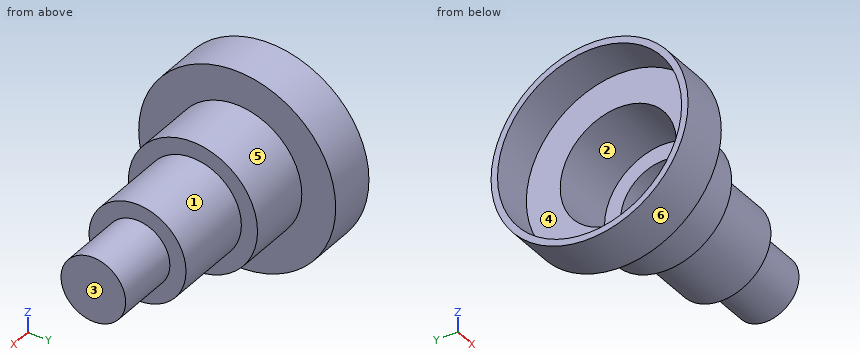
```python
from build123d import *

# Parameters (mm, degrees)
SVUOTA1_T = -2


with BuildPart() as part:
    # Schizzo1 → Rivoluzione1 (revolve)
    with BuildSketch(Plane.XY):
        Polygon((0, 0), (0, 30.5), (15, 30.5), (15, 20), (35, 20), (35, 15), (60, 15), (60, 10), (80, 10), (80, 0), align=None)
    revolve(axis=Axis((80, 0, 0), (-1, 0, 0)))

    # Svuota1
    svuota1_openings = [part.faces().sort_by_distance(p)[0] for p in [
        (0, 0, 0),
    ]]
    offset(amount=SVUOTA1_T, openings=svuota1_openings, kind=Kind.INTERSECTION)


solid = part.part
```
For this review, take the finished solid that the model builds, in its own axes (mm). Face numbers are marked on the shaded views. A direction names the side the tool comes from. Coordinates: 2 decimals unless noted, no trailing zeros. Order: outer loops, then holes, each group sorted by start corner. A loop starts at its lowest first (then second) coordinate and runs counter-clockwise, first axis right, second up. Notation, with made-up numbers: (-35, 27.25) - (13, 27.25) arc R21 cw to (13, 51.25) - close; hole circle Ø9 at (8, 29). An arc over 180 degrees is marked (long way). Answer as a JSON object with one key per item and string values. Group by question number.
1. We need section D-D on z = 11.5. State the section outline as (x, y) points, then the cut area to 3 significant figures.
2. For the marked faces 4, 5 and 6, list the 3-axis set-ups (+Z, -Z, +X, -X, +Y, -Y) from which the entire face can be reached by the end or side of a thin tool; tool diameter is ignored.
3. Clearance check with flat-ended pins moving along their axes: P1, Ø2, axis at y = 12, z = 8, coming from the -X side; P2, Ø5, axis at x = 37, y = -9.5, coming from the +Z side; P3, Ø8, axis at x = 51, y = -0.5, coming from the +Z side; P4, Ø12, axis at x = 54, y = -23.5, coming from the -Z side. State where each tip first meets the part, or that it passes through.
4. The part is to be moulded in two halves that separate along Z. For the marked faces 1, 2 and 3, say which applies: pulls with the +Z half, pulls with the -Z half, needs draft (parallel to the pull), parting line crosses it, or undercut.
5. We need section C-C on x = 36. State the section outline as (y, z) points.
6. For probe 1 along Z at (x, y) = (24, 0); probe 2 along Z at (x, y) = (3.75, 0); probe 3 along X at (y, z) = (24.5, -12), list the stretches that pass through material, from the lowest coordinate up.
Final values:
{
 "1": {"outline": "(0, -28.25) - (15, -28.25) - (15, -16.36) - (35, -16.36) - (35, -9.63) - (60, -9.63) - (60, 9.63) - (35, 9.63) - (35, 16.36) - (15, 16.36) - (15, 28.25) - (0, 28.25) - (0, 26.08) - (13, 26.08) - (13, 13.85) - (33, 13.85) - (33, 6.06) - (58, 6.06) - (58, -6.06) - (33, -6.06) - (33, -13.85) - (13, -13.85) - (13, -26.08) - (0, -26.08) - close", "area": "449 mm²"},
 "2": {"face 4": "-X", "face 5": "+X", "face 6": "+X, -X"},
 "3": {"P1": "x = 33", "P2": "z = 18.33", "P3": "z = 15", "P4": "through"},
 "4": {"face 1": "parting line crosses it", "face 2": "undercut", "face 3": "needs draft"},
 "5": {"outline": "circle Ø30 at (0, 0); hole circle Ø26 at (0, 0)"},
 "6": {"probe 1": "-20 to -18, 18 to 20", "probe 2": "-30.5 to -28.5, 28.5 to 30.5", "probe 3": "13 to 15"}
}
